from build123d import *

# Parameters (mm, degrees)
F0_W     = 40
F0_H     = 70
F1_DEPTH = 600
F3_D     = 11
F3_DEPTH = 50
F4_W     = 40
F4_H     = 30
F5_DEPTH = 90


with BuildPart() as f1:
    # F0 (on Front) → F1 (new body)
    with BuildSketch(Plane.XZ):
        with Locations((20, 35)):
            Rectangle(F0_W, F0_H)
    extrude(amount=F1_DEPTH)

    # F3
    with Locations(Plane.YZ.offset(40)):
        with Locations((-410, 15), (-210, 15)):
            Hole(F3_D / 2, depth=F3_DEPTH)

    # F4 (on face) → F5 (join)
    with BuildSketch(Plane.XZ.offset(600)):
        with Locations((20, 55)):
            Rectangle(F4_W, F4_H)
    extrude(amount=F5_DEPTH)


solid = f1.part
The model under review builds one solid part; all positions refer to its coordinate system, in mm. A direction names the side the tool comes from. Give positions to 0.01 mm unless a question says otherwise; leave off trailing zeros. Write each loop counter-clockwise with the first axis right and the second up, starting at its lowest first coordinate (ties: lowest second). Pieces come first, ordered by that corner, then holes.
1. Tool access review of faces 1 (the flat face through (0, -340, 35)), 2 (the flat face through (20, -644, 40)): name each direction out of +Z, -Z, +X, -X, +Y, -Y from which nothing blocks a thin tool from reaching the whole face with its end or side.
2. For P1, Ø10, axis at x = 8.5, y = -232.5, coming from the -Z side; P2, Ø9, axis at y = -210, z = 15, coming from the -X side; P3, Ø1.5, axis at x = 21.5, z = 21, coming from the -Y side, all flat-tipped, find the tip position at first contact; note any pin that passes through.
3. Wall thickness on L1, parallel to Z at x = 30, y = -210; L2, parallel to Y at x = 2, z = 17; L3, parallel to Y at x = 30, z = 23: over which ranges is each line inside the solid? List them lowest first.
4. Draft analysis for pull direction Y (two halves, no side actions). For faces 3 (the cylindrical face through (19.72, -204.505, 15.242)), 4 (the flat face through (20, -296, 0)), 5 (the cylindrical face through (19.72, -415.246, 16.652)), 6 (the flat face through (20, 0, 35)), state which applies: +Y half, -Y half, draft (parallel to the pull), parting line (faces both ways), or undercut.
5. Add section A-A, the plane x = 22. Write out the cut boundary in (y, z), plus the area to 3 significant figures.
Worked answers:
1. face 1: +Z, -Z, -X, +Y, -Y
1. face 2: -Z, +X, -X, -Y
2. P1: stops at z = 0
2. P2: passes through
2. P3: stops at y = -600
3. L1: z = 0 to 9.5, 20.5 to 70
3. L2: y = -600 to -415.12, -404.88 to -215.12, -204.88 to 0
3. L3: y = -600 to 0
4. face 3: undercut
4. face 4: draft
4. face 5: undercut
4. face 6: +Y half
5. outline: (-690, 40) - (-600, 40) - (-600, 0) - (0, 0) - (0, 70) - (-690, 70) - close; hole circle Ø11 at (-410, 15); hole circle Ø11 at (-210, 15)
5. area: 44,500 mm2
